Source: CAD feature listing. Evaluate the final solid. Frame: model axes, mm. Round coordinates to 2 decimals unless told otherwise and drop trailing zeros. One line per question, with ' | ' between items.
from build123d import *

# Parameters (mm, degrees)
SKETCH_1_W          = 45
SKETCH_1_H          = 45
EXTRUDE_1_DEPTH     = 150
SKETCH_2_W          = 45
SKETCH_2_H          = 45
EXTRUDE_2_DEPTH     = 10
SKETCH_5_R          = 3
CUT_EXTRUDE_1_DEPTH = 30
FILLET_1_R          = 3


with BuildPart() as part:
    # 草图1 → 凸台-拉伸1 (new body)
    with BuildSketch(Plane(origin=(0, 0, 0), x_dir=(1, 0, 0), z_dir=(0, 1, 0))):
        Rectangle(SKETCH_1_W, SKETCH_1_H)
    extrude(amount=EXTRUDE_1_DEPTH)

    # 草图3 for 放样1 → 放样1 section 0
    with BuildSketch(Plane(origin=(0, 175, 0), x_dir=(1, 0, 0), z_dir=(0, 1, 0))):
        with BuildLine():
            # circular arc as an exact rational Bezier (weights 1, cos(half-angle), 1)
            Bezier((7.071067812, -7.071067812), (14.142135623, 0), (7.071067812, 7.071067812), weights=[1, 0.707106781, 1])
            Bezier((7.071067812, 7.071067812), (0, 14.142135623), (-7.071067812, 7.071067812), weights=[1, 0.707106781, 1])
            Bezier((-7.071067812, 7.071067812), (-14.142135623, 0), (-7.071067812, -7.071067812), weights=[1, 0.707106781, 1])
            Bezier((-7.071067812, -7.071067812), (0, -14.142135623), (7.071067812, -7.071067812), weights=[1, 0.707106781, 1])
        make_face()
    # 草图2 → 放样1 section 1
    with BuildSketch(Plane(origin=(0, 150, 0), x_dir=(1, 0, 0), z_dir=(0, 1, 0))):
        Rectangle(SKETCH_2_W, SKETCH_2_H)
    loft()

    # 草图4 → 凸台-拉伸2 (add)
    with BuildSketch(Plane(origin=(0, 175, 0), x_dir=(1, 0, 0), z_dir=(0, 1, 0))):
        with BuildLine():
            ThreePointArc((-7.071067812, 7.071067812), (-10, 0), (-7.071067812, -7.071067812))
            ThreePointArc((-7.071067812, -7.071067812), (0, -10), (7.071067812, -7.071067812))
            ThreePointArc((7.071067812, -7.071067812), (10, 0), (7.071067812, 7.071067812))
            ThreePointArc((7.071067812, 7.071067812), (0, 10), (-7.071067812, 7.071067812))
        make_face()
    extrude(amount=EXTRUDE_2_DEPTH)

    # 草图5 → 切除-拉伸1 (cut)
    with BuildSketch(Plane(origin=(0, 185, 0), x_dir=(1, 0, 0), z_dir=(0, 1, 0))):
        with Locations(Location((0, 0, 0), (0, 0, 270))):
            Circle(SKETCH_5_R)
    extrude(amount=-CUT_EXTRUDE_1_DEPTH, mode=Mode.SUBTRACT)

    # 圆角1
    fillet_1_edges = [part.edges().sort_by_distance(p)[0] for p in [
        (22.5, 75, -22.5),
        (22.5, 75, 22.5),
        (-22.5, 75, -22.5),
        (-22.5, 75, 22.5),
    ]]
    fillet(fillet_1_edges, radius=FILLET_1_R)


solid = part.part
1. Contact query for a flat-ended pin moving along its axis: P1, Ø5, axis at x = 0, z = 0, coming from the +Y side. Output: stop coordinate, or through.
Worked out:
P1: stops at y = 155
2. Mould query, pull axis X, two halves, no side actions, for faces 1 (the cylindrical face through (0.9, 170.21, 2.86)), 2 (the flat face through (0, 155, 0)), 3 (the cylindrical face through (-21.64, 76.77, 21.6)), 4 (the flat face through (0, 74, 22.5)). Classes: released by +X, released by -X, zero draft, split by the parting line, or undercut.
Worked out:
face 1: undercut | face 2: undercut | face 3: released by -X | face 4: zero draft
3. Material intervals for probe 1 along X at (y, z) = (174, 0); probe 2 along X at (y, z) = (164, 0); probe 3 along Y at (x, z) = (-12.5, -2), sorted ascending.
Worked out:
probe 1: x = -10.5 to -3, 3 to 10.5 | probe 2: x = -15.5 to -3, 3 to 15.5 | probe 3: y = 0 to 169.83
